```python
from build123d import *

# Parameters (mm, degrees)
F1_DEPTH = 63.5
F2_DEPTH = 25.4
F3_DEPTH = 7.9375
F0_W     = 25.4
F0_H     = 19.05
F4_DEPTH = 25.4
F6_R     = 6.35


# Not quite as in the source:
# - a feature names something its author has since deleted; it is built from what else it names


with BuildPart() as f1:
    # F0 (on Front) → F1 (new body, symmetric)
    with BuildSketch(Plane.XZ):
        Polygon((-41.275, 9.525), (-41.275, -9.525), (41.275, -9.525), (41.275, 9.525), (22.225, 9.525), align=None)
    extrude(amount=F1_DEPTH, both=True)

    # F0 (on Front) → F2 (join, symmetric)
    with BuildSketch(Plane.XZ):
        with BuildLine():
            Line((22.225, 9.525), (41.275, 9.525))
            Line((41.275, 9.525), (41.275, 27.0002))
            ThreePointArc((41.275, 27.0002), (45.9246798487, 38.2255201513), (57.15, 42.8752))
            Line((57.15, 42.8752), (60.325, 42.8752))
            Line((60.325, 42.8752), (60.325, 61.9252))
            Line((60.325, 61.9252), (57.15, 61.9252))
            add(Edge.make_bspline(
                [(48.8367454286, 60.9213648301), (51.9709953624, 61.5161426584), (54.7763944368, 61.8635493609), (57.15, 61.9252)],
                knots=[100.9548457495, 100.9548457495, 100.9548457495, 100.9548457495, 111.5045361635, 111.5045361635, 111.5045361635, 111.5045361635], degree=3))
            ThreePointArc((48.8367454286, 60.9213648301), (29.6718628642, 48.5572778295), (22.225, 27.0002))
            Line((22.225, 27.0002), (22.225, 9.525))
        make_face()
    extrude(amount=F2_DEPTH, both=True)

    # F0 (on Front) → F3 (join, symmetric)
    with BuildSketch(Plane.XZ):
        with BuildLine():
            add(Edge.make_bspline(
                [(-41.275, 9.525), (-41.2637939453, 26.8850534088), (18.8436644761, 55.2296618934), (48.8367454286, 60.9213648301)],
                knots=[0, 0, 0, 0, 100.9548457495, 100.9548457495, 100.9548457495, 100.9548457495], degree=3))
            Line((-41.275, 9.525), (22.225, 9.525))
            Line((22.225, 9.525), (22.225, 27.0002))
            ThreePointArc((22.225, 27.0002), (29.6718628642, 48.5572778295), (48.8367454286, 60.9213648301))
        make_face()
    extrude(amount=F3_DEPTH, both=True)

    # F0 (on Front) → F4 (join, symmetric)
    with BuildSketch(Plane.XZ):
        with Locations((73.025, 52.4002)):
            Rectangle(F0_W, F0_H)
    extrude(amount=F4_DEPTH, both=True)

    # F0 (on Front) → F5 (revolve)
    with BuildSketch(Plane.XZ):
        Polygon((85.725, 66.675), (85.725, 61.9252), (85.725, 42.8752), (85.725, 38.1), (111.125, 38.1), (111.125, 66.675), align=None)
    revolve(axis=Axis((85.725, 0, 52.3875), (0, 0, 1)))

    # F6
    f6_edges = [f1.edges().sort_by_distance(p)[0] for p in [
        (41.275, 63.5, 0),
        (41.275, -63.5, 0),
        (-41.275, -63.5, 0),
        (-41.275, 63.5, 0),
    ]]
    fillet(f6_edges, radius=F6_R)


solid = f1.part
```
Input: part model. Units: mm. Frame: model coordinates. A direction names the side the tool comes from. Coordinates: 2 decimals unless noted, no trailing zeros. Write each loop counter-clockwise with the first axis right and the second up, starting at its lowest first coordinate (ties: lowest second). Pieces come first, ordered by that corner, then holes. Notation, with made-up numbers: (43, -9.5) - (88, -9.5) arc R15 ccw to (88, 10.5) - close; hole circle Ø3 at (43, 52). An arc over 180 degrees is marked (long way). Put each result on its own line as item: value. Start each with the question number.
1) Reachability of faces 1 (the face through (-6, 7.938, 24)), 2 (the face through (46, -25.4, 42)), 3 (the face through (46, 25.4, 42)), 4 (the face through (60, 2, 61.925)), 5 (the face through (60, 2, 42.875)) from +Z, -Z, +X, -X, +Y, -Y: full face, straight path, thin tool, end or side. Return the list, or none.
2) Cut plane D-D (x = 100.5). Return the cut outline in (y, z) (3 decimals), plus the area to 3 significant figures.
3) Ray query, L1, parallel to X at y = -13.5, z = 12 (3 decimals); L2, parallel to Z at x = 68.5, y = 7 (3 decimals); L3, parallel to Y at x = 5.5, z = 28. Return the intervals inside material, ascending.
4) Contact query for flat-ended pins moving along their axis: pin 1 (1.5 mm diameter, centred on y = -10, z = 29.5, fed in from +X); pin 2 (5 mm diameter, centred on y = -13, z = 14, fed in from -X) (3 decimals); pin 3 (15.5 mm diameter, centred on x = 46.5, z = 48, fed in from +Y). Output: stop coordinate, or through.
5) Cut plane A-A (z = -0.5). Return the cut outline in (x, y) (3 decimals), plus the area to 3 significant figures.
6) Cut plane B-B (x = 63.5). Return the cut outline in (y, z) (3 decimals), plus the area to 3 significant figures.
7) Cut plane C-C (y = 48.5). Return the cut outline in (x, z) (3 decimals), plus the area to 3 significant figures.
Resolved:
1. face 1: +Z, -X, +Y
1. face 2: +Z, +X, -X, -Y
1. face 3: +Z, +X, -X, +Y
1. face 4: +Z, -X
1. face 5: -Z
2. outline: (-20.661, 38.1) - (20.661, 38.1) - (20.661, 66.675) - (-20.661, 66.675) - close
2. area: 1,180 mm2
3. L1: x = 22.225 to 41.275
3. L2: z = 38.1 to 66.675
3. L3: y = -7.94 to 7.94
4. pin 1: stops at x = 41.61
4. pin 2: stops at x = 22.225
4. pin 3: stops at y = 25.4
5. outline: (-41.275, -57.15) arc R6.35 ccw to (-34.925, -63.5) - (34.925, -63.5) arc R6.35 ccw to (41.275, -57.15) - (41.275, 57.15) arc R6.35 ccw to (34.925, 63.5) - (-34.925, 63.5) arc R6.35 ccw to (-41.275, 57.15) - close
5. area: 10,400 mm2
6. outline: (-25.4, 42.875) - (-12.297, 42.875) - (-12.297, 38.1) - (12.297, 38.1) - (12.297, 42.875) - (25.4, 42.875) - (25.4, 61.925) - (12.297, 61.925) - (12.297, 66.675) - (-12.297, 66.675) - (-12.297, 61.925) - (-25.4, 61.925) - close
6. area: 1,200 mm2
7. outline: (-41.275, -9.525) - (41.275, -9.525) - (41.275, 9.525) - (-41.275, 9.525) - close
7. area: 1,570 mm2
